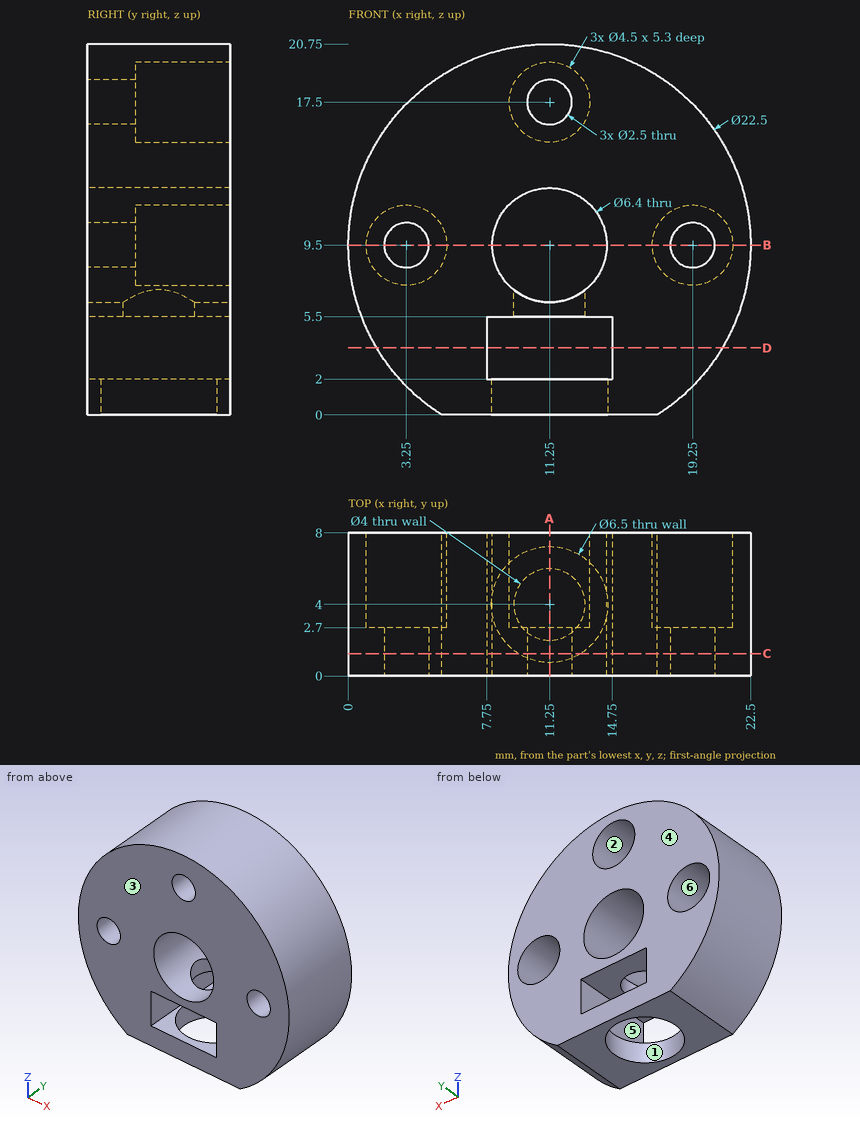
Can you work these out from the drawing? Everything is in mm from the part's minimum corner. A direction names the side the tool comes from. Coordinates: 2 decimals unless noted, no trailing zeros. Loops run counter-clockwise (first coordinate to the right, second up) from the corner with the lowest first, then second, coordinate; pieces in that order, holes last.
1) Thinking about a two-plate mould opening in Y: for the marked faces 1, 2 and 3, which applies, released by +Y, released by -Y, zero draft, split by the parting line, or undercut?
Reported:
face 1: undercut
face 2: zero draft
face 3: released by -Y
2) Imagine slicing it at A-A (x = 11.25). List the corners of the cut face in (y, z) for me, and give its area (3 significant figures).
Reported:
outline: (0, 0) - (0.75, 0) - (0.75, 2) - (0, 2) - close; (0, 5.5) - (2, 5.5) - (2, 6.3) - (0, 6.3) - close; (0, 12.7) - (8, 12.7) - (8, 15.25) - (2.7, 15.25) - (2.7, 16.25) - (0, 16.25) - close; (0, 18.75) - (2.7, 18.75) - (2.7, 19.75) - (8, 19.75) - (8, 20.75) - (0, 20.75) - close; (6, 5.5) - (8, 5.5) - (8, 6.3) - (6, 6.3) - close; (7.25, 0) - (8, 0) - (8, 2) - (7.25, 2) - close
area: 40.0 mm2
3) Imagine slicing it at B-B (z = 9.5). List the corners of the cut face in (x, y) for me, and give its area (3 significant figures).
Reported:
outline: (0, 0) - (2, 0) - (2, 2.7) - (1, 2.7) - (1, 8) - (0, 8) - close; (4.5, 0) - (8.05, 0) - (8.05, 8) - (5.5, 8) - (5.5, 2.7) - (4.5, 2.7) - close; (14.45, 0) - (18, 0) - (18, 2.7) - (17, 2.7) - (17, 8) - (14.45, 8) - close; (20.5, 0) - (22.5, 0) - (22.5, 8) - (21.5, 8) - (21.5, 2.7) - (20.5, 2.7) - close
area: 67.6 mm2
4) Imagine slicing it at D-D (z = 3.75). List the corners of the cut face in (x, y) for me, and give its area (3 significant figures).
Reported:
outline: (1.58, 0) - (7.75, 0) - (7.75, 8) - (1.58, 8) - close; (14.75, 0) - (20.92, 0) - (20.92, 8) - (14.75, 8) - close
area: 98.7 mm2
5) Imagine slicing it at C-C (y = 1.25). List the corners of the cut face in (x, z) for me, and give its area (3 significant figures).
Reported:
outline: (5.22, 0) - (9.52, 0) - (9.52, 2) - (7.75, 2) - (7.75, 5.5) - (14.75, 5.5) - (14.75, 2) - (12.98, 2) - (12.98, 0) - (17.28, 0) arc R11.25 ccw (long way) to start; hole circle Ø2.5 at (3.25, 9.5); hole circle Ø6.4 at (11.25, 9.5); hole circle Ø2.5 at (11.25, 17.5); hole circle Ø2.5 at (19.25, 9.5)
area: 305 mm2
6) Will these pins go through, and if not, where does the flat tip stop? pin 1 Ø1.3 at (x, z) = (4, 10.5) entering from +Y; pin 2 Ø4 at (y, z) = (1.5, 18.5) entering from +X; pin 3 Ø1.8 at (y, z) = (5, 4) entering from -X.
Reported:
pin 1: stops at y = 2.7
pin 2: stops at x = 20.06
pin 3: stops at x = 0.98
7) Please list where these lines run through material, in increasing order: line 1 along Z through (x, y) = (13.75, 0.75); line 2 along X through (y, z) = (5.5, 8); line 3 along Y through (x, z) = (11.25, 5.8).
Reported:
line 1: z = 0 to 2, 5.5 to 7.5, 11.5 to 20.47
line 2: x = 0.1 to 1.57, 4.93 to 8.42, 14.08 to 17.57, 20.93 to 22.4
line 3: y = 0 to 2, 6 to 8
8) Which directions (+Z, -Z, +X, -X, +Y, -Y) give clear straight access to the entire face, cutting with the end or side of a thin tool? Please do the marked faces 4, 5 and 6.
Reported:
face 4: +Z, -Z, +X, -X, +Y
face 5: +Y, -Y
face 6: +Y
